```python
from build123d import *

# Parameters (mm, degrees)
SKETCH_R     = 1.65
PAD_DEPTH    = 7
SKETCH001_W  = 40
SKETCH001_H  = 2
PAD001_DEPTH = 20
FILLET_R     = 3
FILLET001_R  = 10
SKETCH002_R  = 1.55
POCKET_DEPTH = 5
SKETCH003_R  = 1.5
PAD002_DEPTH = 5
FILLET002_R  = 1
FILLET003_R  = 1
FILLET004_R  = 0.5


with BuildPart() as part:
    # Sketch → Pad (new body)
    with BuildSketch(Plane.XY):
        with BuildLine():
            Line((0, 0), (20, 0))
            Line((20, 0), (20, 3.45))
            Line((18.999985, 3.45), (20, 3.45))
            ThreePointArc((18.999985, 6.55), (17.45, 5), (18.999985, 3.45))
            Line((18.999985, 6.55), (20, 6.55))
            Line((20, 6.55), (20, 8.164485))
            Line((14, 8.164485), (20, 8.164485))
            ThreePointArc((14, 11.764485), (12.2, 9.964485), (14, 8.164485))
            Line((14, 11.764485), (20, 11.764485))
            Line((20, 11.764485), (20, 13.45))
            Line((19, 13.45), (20, 13.45))
            ThreePointArc((19, 16.55), (17.45, 15), (19, 13.45))
            Line((19, 16.55), (20, 16.55))
            Line((20, 16.55), (20, 20))
            Line((20, 20), (0, 20))
            Line((0, 20), (0, 0))
        make_face()
        with Locations((4, 10)):
            Circle(SKETCH_R, mode=Mode.SUBTRACT)
    extrude(amount=PAD_DEPTH)

    # Sketch001 → Pad001 (new body)
    with BuildSketch(Plane(origin=(0, 20, 0), x_dir=(-1, 0, 0), z_dir=(0, 1, 0))):
        with Locations((-20, 6)):
            Rectangle(SKETCH001_W, SKETCH001_H)
    extrude(amount=PAD001_DEPTH)

    # Fillet
    fillet_edges = [part.edges().sort_by_distance(p)[0] for p in [
        (40, 20, 6),
        (40, 40, 6),
        (0, 40, 6),
    ]]
    fillet(fillet_edges, radius=FILLET_R)

    # Fillet001
    fillet001_edges = [part.edges().sort_by_distance(p)[0] for p in [
        (0, 20, 2.5),
    ]]
    fillet(fillet001_edges, radius=FILLET001_R)

    # Sketch002 → Pocket (cut)
    with BuildSketch(Plane.XY.offset(7)):
        with Locations((20, 25)):
            Circle(SKETCH002_R)
    extrude(amount=-POCKET_DEPTH, mode=Mode.SUBTRACT)

    # Sketch003 → Pad002 (new body)
    with BuildSketch(Plane(origin=(0, 0, 5), x_dir=(1, 0, 0), z_dir=(0, 0, -1))):
        with Locations((35, -35)):
            Circle(SKETCH003_R)
    extrude(amount=PAD002_DEPTH)

    # Fillet002
    fillet002_edges = [part.edges().sort_by_distance(p)[0] for p in [
        (33.5, 35, 0),
    ]]
    fillet(fillet002_edges, radius=FILLET002_R)

    # Fillet003
    fillet003_edges = [part.edges().sort_by_distance(p)[0] for p in [
        (2.35, 10, 0),
    ]]
    fillet(fillet003_edges, radius=FILLET003_R)

    # Fillet004
    fillet004_edges = [part.edges().sort_by_distance(p)[0] for p in [
        (17.45, 5, 0),
        (19.499993, 3.45, 0),
        (19.499993, 6.55, 0),
        (17, 8.164485, 0),
        (12.2, 9.964485, 0),
        (17, 11.764485, 0),
        (19.5, 13.45, 0),
        (17.45, 15, 0),
        (19.5, 16.55, 0),
        (19.5, 16.55, 7),
        (17.45, 15, 7),
        (19.5, 13.45, 7),
        (17, 11.764485, 7),
        (12.2, 9.964485, 7),
        (17, 8.164485, 7),
        (19.499993, 6.55, 7),
        (17.45, 5, 7),
        (19.499993, 3.45, 7),
    ]]
    fillet(fillet004_edges, radius=FILLET004_R)


solid = part.part
```
Build history of the part. All positions in model axes, mm. A direction names the side the tool comes from. Coordinates: 2 decimals unless noted, no trailing zeros. Order: outer loops, then holes, each group sorted by start corner. A loop starts at its lowest first (then second) coordinate and runs counter-clockwise, first axis right, second up. Notation, with made-up numbers: (16, 34) -> (40, 34) arc R24 ccw to (40, 55) -> close; hole circle Ø9 at (15.25, -0.75). An arc over 180 degrees is marked (long way). Answer in a Markdown table with one row per item. Add a question column.
Q1. Drop flat-ended pins along their axis: pin 1 (0.5 mm diameter, centred on x = 19.5, z = 2.5, fed in from +Y); pin 2 (0.8 mm diameter, centred on x = 19.5, z = 4, fed in from -Y); pin 3 (4 mm diameter, centred on y = 17.5, z = 2.5, fed in from +X); pin 4 (1.5 mm diameter, centred on x = 30, z = 5.5, fed in from -Y). Give the stop position or say it passes through.
Q2. Wall check: line 1 along Y through (x, z) = (19, 2); line 2 along X through (y, z) = (2, 3.5); line 3 along Y through (x, z) = (19, 6.25). Give the ranges that are in metal, low to high. Write a range as [from, to].
Q3. Mould opens along Y. For faces 6 (the face through (17.45, 15.03, 3.46)), 7 (the face through (39.14, 20.9, 6.01)), 8 (the face through (3.01, 17.15, 2.54)) say: +Y half, -Y half, draft (parallel to the pull), parting line (faces both ways), or undercut.
Q4. Band-saw the part on D-D, the plane y = 15. List the corners of the cut face in (x, z).
Q5. Band-saw the part on C-C, the plane z = 6. List the corners of the cut face in (x, y).
Q6. Band-saw the part on B-B, the plane y = 25. List the corners of the cut face in (x, z), then the cut area to 3 significant figures.
Q7. Band-saw the part on A-A, the plane x = 4. List the corners of the cut face in (y, z).
Q8. Which spindle directions (+Z, -Z, +X, -X, +Y, -Y) get a long thin tool onto all of the face, cutting with end or side? Do faces 1 (the face through (19.798, 26.537, 6.014)), 2 (the face through (20, 2, 3)), 3 (the face through (17, 11.764, 3)), 4 (the face through (33.8, 35.9, 3)), 5 (the face through (40, 30, 6)). Say none if no direction does.
Answers follow:
| question | item | result |
|---|---|---|
| 1 | pin 1 | y = 20 |
| 1 | pin 2 | y = 0 |
| 1 | pin 3 | x = 20 |
| 1 | pin 4 | y = 20 |
| 2 | line 1 | [0, 3.45], [6.55, 8.16], [11.76, 13.45], [16.55, 20] |
| 2 | line 2 | [0, 20] |
| 2 | line 3 | [0, 3.45], [6.55, 8.16], [11.76, 13.45], [16.55, 23.82], [26.18, 40] |
| 3 | face 6 | undercut |
| 3 | face 7 | -Y half |
| 3 | face 8 | +Y half |
| 4 | outline | (0, 5) -> (1.34, 5) -> (1.34, 0) -> (16.95, 0) arc R0.5 ccw to (17.45, 0.5) -> (17.45, 6.5) arc R0.5 ccw to (16.95, 7) -> (0, 7) -> close |
| 5 | outline | (0, 0) -> (20, 0) -> (20, 3.45) -> (19, 3.45) arc R1.55 cw to (19, 6.55) -> (20, 6.55) -> (20, 8.16) -> (14, 8.16) arc R1.8 cw to (14, 11.76) -> (20, 11.76) -> (20, 13.45) -> (19, 13.45) arc R1.55 cw to (19, 16.55) -> (20, 16.55) -> (20, 20) -> (37, 20) arc R3 ccw to (40, 23) -> (40, 37) arc R3 ccw to (37, 40) -> (3, 40) arc R3 ccw to (0, 37) -> close; hole circle Ø3.3 at (4, 10); hole circle Ø3.1 at (20, 25) |
| 6 | outline | (0, 5) -> (18.45, 5) -> (18.45, 7) -> (0, 7) -> close; (21.55, 5) -> (40, 5) -> (40, 7) -> (21.55, 7) -> close |
| 6 | area | 73.8 mm^2 |
| 7 | outline | (0, 0) -> (7.35, 0) arc R1 ccw to (8.35, 1) -> (8.35, 7) -> (0, 7) -> close; (11.65, 1) arc R1 ccw to (12.65, 0) -> (18, 0) -> (18, 5) -> (40, 5) -> (40, 7) -> (11.65, 7) -> close |
| 8 | face 1 | +Z, -Z |
| 8 | face 2 | +Z, -Z, +X, -Y |
| 8 | face 3 | +Z, -Z, +X |
| 8 | face 4 | -Z |
| 8 | face 5 | +Z, -Z, +X, +Y, -Y |
